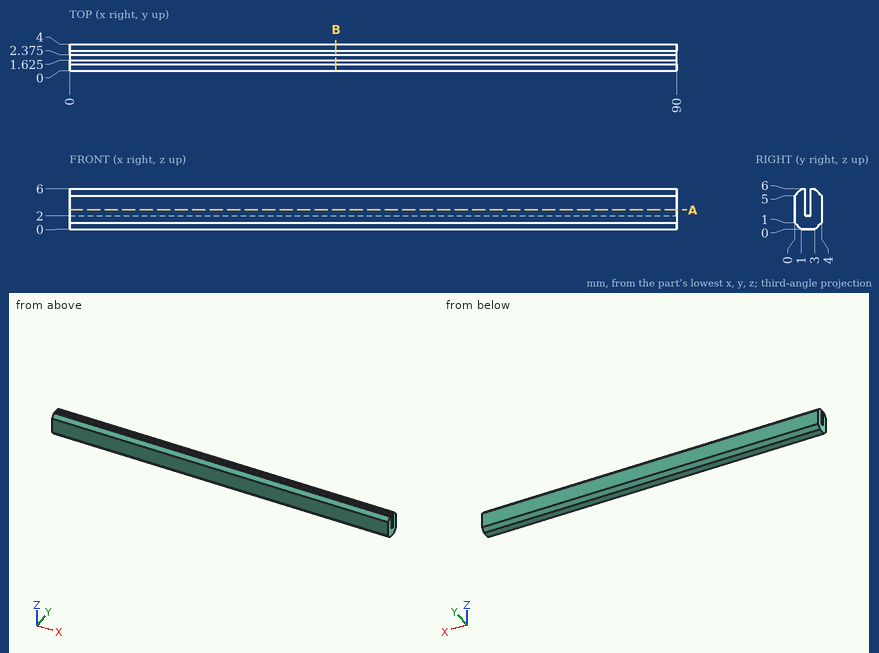
Source: three-view drawing plus pictorial views. Frame: mm from the lowest corner of the part. Give positions to 0.01 mm unless a question says otherwise; leave off trailing zeros. Loops run counter-clockwise (first coordinate to the right, second up) from the corner with the lowest first, then second, coordinate; pieces in that order, holes last. Notation, with made-up numbers: M -24.5,-13.5 L -3.5,-13.5 A9 cw -3.5,2.5 Z; hole C 30.25,35.25 d2. An arc over 180 degrees is marked long. Use CSV: the item, a comma, the result in double quotes.
(1) Material intervals for L1, parallel to Y at x = 79, z = 2.95 (3 decimals); L2, parallel to Z at x = 50, y = 2.1; L3, parallel to Y at x = 69.5, z = 0.7, sorted ascending. Write a range as [from, to].
Outcome:
L1,"y = [0, 1.625], [2.375, 4]"
L2,"z = [0, 2]"
L3,"y = [0.3, 3.7]"
(2) Section B-B, the plane x = 39.5. Return loops of the section in (y, z) (3 decimals).
Outcome:
outline,"M 0,1 L 1,0 L 3,0 L 4,1 L 4,5 L 3,6 L 2.375,6 L 2.375,2 L 1.625,2 L 1.625,6 L 1,6 L 0,5 Z"
(3) Section A-A, the plane z = 2.9. Return loops of the section in (x, y) (3 decimals).
Outcome:
outline,"M 0,0 L 90,0 L 90,1.625 L 0,1.625 Z; M 0,2.375 L 90,2.375 L 90,4 L 0,4 Z"
